Can you work these out from the model? Positions are in its coordinate system, mm. A direction names the side the tool comes from. Give positions to 0.01 mm unless a question says otherwise; leave off trailing zeros. Write each loop counter-clockwise with the first axis right and the second up, starting at its lowest first coordinate (ties: lowest second). Pieces come first, ordered by that corner, then holes. Notation, with made-up numbers: M 17,59 L 43,59 A14 cw 43,86 Z; hole C -9.75,55 d6. An arc over 180 degrees is marked long. Answer as CSV lines item,"result". Start each with the question number.
```python
from build123d import *

# Parameters (mm, degrees)
BOSS_EXTRUDE1_DEPTH = 22.5
SKETCH2_R           = 16.25
CUT_EXTRUDE1_DEPTH  = 10
SKETCH3_R           = 7
CUT_EXTRUDE2_DEPTH  = 25
SKETCH4_R           = 1.5
CUT_EXTRUDE4_DEPTH  = 10


with BuildPart() as part:
    # Sketch1 → Boss-Extrude1 (new, symmetric)
    with BuildSketch(Plane.XY):
        Polygon((-17.5, 30.310889132), (17.5, 30.310889132), (35, 0), (17.5, -30.310889132), (-17.5, -30.310889132), (-35, 0), align=None)
    extrude(amount=BOSS_EXTRUDE1_DEPTH, both=True)

    # Sketch2 → Cut-Extrude1 (cut)
    with BuildSketch(Plane.XY.offset(22.5)):
        Circle(SKETCH2_R)
    cut_extrude1 = extrude(amount=-CUT_EXTRUDE1_DEPTH, mode=Mode.SUBTRACT)

    # Mirror1: Cut-Extrude1 across plane
    add(cut_extrude1.mirror(Plane.XY), mode=Mode.SUBTRACT)

    # Sketch3 → Cut-Extrude2 (cut)
    with BuildSketch(Plane(origin=(0, 0, -12.5), x_dir=(-1, 0, 0), z_dir=(0, 0, -1))):
        Circle(SKETCH3_R)
    extrude(amount=-CUT_EXTRUDE2_DEPTH, mode=Mode.SUBTRACT)

    # Sketch4 → Cut-Extrude4 (cut)
    with BuildSketch(Plane.XY.offset(22.5)):
        with Locations((0, 20)):
            Circle(SKETCH4_R)
    cut_extrude4 = extrude(amount=-CUT_EXTRUDE4_DEPTH, mode=Mode.SUBTRACT)

    # Mirror2: Cut-Extrude4 across plane
    add(cut_extrude4.mirror(Plane.XY), mode=Mode.SUBTRACT)


solid = part.part
```
1) I need wall thicknesses on L1, parallel to Y at x = 0, z = 16; L2, parallel to Y at x = 0, z = -0.5; L3, parallel to X at y = 4, z = -0.5. Which ranges of each line are inside material? Lowest first, please. Write a range as from..to.
2) I want a section at C-C, the plane z = -9.5. Please give me the cut outline in (x, y), then the cut area to 3 significant figures.
3) I'm going to push flat-ended pins straight in: P1, Ø1.5, axis at y = 15, z = 4.5, coming from the +X side; P2, Ø16, axis at x = -6, y = 5.5, coming from the -Z side; P3, Ø10, axis at y = 6.5, z = 2.5, coming from the +X side. Where does each tip first touch, or does it pass through?
4) I want a section at A-A, the plane z = 13.5. Please give me the cut outline in (x, y).
5) I want a section at D-D, the plane y = 20. Please give me the cut outline in (x, z).
6) On a 3-axis mill with a long thin cutter (end or side, diameter ignored), from which of +Z, -Z, +X, -X, +Y, -Y can I reach the whole of each face in a straight line? I mean faces 5 (the flat face through (-26.372, 14.943, 0.315)), 6 (the flat face through (0, 20, 12.5)), 7 (the cylindrical face through (-0.195, 21.487, -17.57)). Say none if no direction works.
7) I want a section at B-B, the plane x = 0. Please give me the cut outline in (y, z).
8) Thinking about a two-plate mould opening in Y: for faces 1 (the flat face through (7, -3, -12.5)), 2 (the flat face through (-26.128, -15.368, 0.315)), 3 (the flat face through (-15, 7, 22.5)), 4 (the flat face through (0, 30.311, 0)), which applies, released by +Y, released by -Y, zero draft, split by the parting line, or undercut?
Values found:
1,L1,"y = -30.31..-16.25, 16.25..18.5, 21.5..30.31"
1,L2,"y = -30.31..-7, 7..30.31"
1,L3,"x = -32.69..-5.74, 5.74..32.69"
2,outline,"M -35,0 L -17.5,-30.31 L 17.5,-30.31 L 35,0 L 17.5,30.31 L -17.5,30.31 Z; hole C 0,0 d14"
2,area,"3,030 mm²"
3,P1,"stops at x = 26.77"
3,P2,"stops at z = -12.5"
3,P3,"stops at x = 34.13"
4,outline,"M -35,0 L -17.5,-30.31 L 17.5,-30.31 L 35,0 L 17.5,30.31 L -17.5,30.31 Z; hole C 0,0 d32.5; hole C 0,20 d3"
5,outline,"M -23.45,-22.5 L -1.5,-22.5 L -1.5,-12.5 L 1.5,-12.5 L 1.5,-22.5 L 23.45,-22.5 L 23.45,22.5 L 1.5,22.5 L 1.5,12.5 L -1.5,12.5 L -1.5,22.5 L -23.45,22.5 Z"
6,face 5,"+Z, -Z, -X, +Y"
6,face 6,"+Z"
6,face 7,"-Z"
7,outline,"M -30.31,-22.5 L -16.25,-22.5 L -16.25,-12.5 L -7,-12.5 L -7,12.5 L -16.25,12.5 L -16.25,22.5 L -30.31,22.5 Z; M 7,-12.5 L 16.25,-12.5 L 16.25,-22.5 L 18.5,-22.5 L 18.5,-12.5 L 21.5,-12.5 L 21.5,-22.5 L 30.31,-22.5 L 30.31,22.5 L 21.5,22.5 L 21.5,12.5 L 18.5,12.5 L 18.5,22.5 L 16.25,22.5 L 16.25,12.5 L 7,12.5 Z"
8,face 1,"undercut"
8,face 2,"released by -Y"
8,face 3,"zero draft"
8,face 4,"released by +Y"
